Here's how the part is built. I have some questions about the finished solid (model axes, mm). A direction names the side the tool comes from. Give positions to 0.01 mm unless a question says otherwise; leave off trailing zeros. Write each loop counter-clockwise with the first axis right and the second up, starting at its lowest first coordinate (ties: lowest second). Pieces come first, ordered by that corner, then holes. Notation, with made-up numbers: (70.25, -38.5) - (86.25, -38.5) arc R27 ccw to (86.25, -2.5) - close; hole circle Ø1 at (89, 81). An arc over 180 degrees is marked (long way). Use one line per item in the form item = value. Start each with the question number.
Solid Edge part; units mm, degrees
sketch "Sketch1" plane through (0, 0, 0) normal (0, -1, 0) x (1, 0, 0)
  line L0 (0, 50) -> (4, 50)
  arc A0 (4, 50) -> (28, 78) centre (31.9985, 50.287) cw
  line L1 (28, 50) -> (28, 78)
  line L2 (28, 35) -> (28, 50)
  line L3 (152, 35) -> (28, 35)
  line L4 (152, 51) -> (152, 35)
  line L5 (180, 51) -> (152, 51)
  line L6 (180, 0) -> (180, 51)
  line L7 (0, 0) -> (180, 0)
  line L8 (0, 0) -> (0, 50)
extrude "Protrusion1" add sketch "Sketch1" against normal blind 70
sketch "Sketch2" plane through (180, 35, 25.5) normal (1, 0, 0) x (0, 1, 0)
  circle A0 centre (0, 25.5) radius 16
extrude "ExtrudedProtrusion_2" add sketch "Sketch2" against normal blind 28
sketch "Sketch3" plane through (180, 35, 33.5) normal (1, 0, 0) x (0, 1, 0)
  circle A0 centre (0, 17.5) radius 8
extrude "ExtrudedCutout_1" cut sketch "Sketch3" against normal blind 28 and the other way blind 1
sketch "Sketch4" plane through (180, 35, 33.5) normal (1, 0, 0) x (0, 1, 0)
  line L0 (16, -33.5) -> (16, -14.5)
  line L1 (16, -14.5) -> (8, -14.5)
  line L2 (8, -14.5) -> (8, 7.5)
  line L3 (8, 7.5) -> (-8, 7.5)
  line L4 (-8, 7.5) -> (-8, -14.5)
  line L5 (-8, -14.5) -> (-16, -14.5)
  line L6 (-16, -14.5) -> (-16, -33.5)
  line L7 (-16, -33.5) -> (16, -33.5)
extrude "ExtrudedCutout_2" cut sketch "Sketch4" against normal blind 180 and the other way blind 1
1. Please list where these lines run through material, in increasing order: line 1 (Z direction, x = 169, y = 35); line 2 (X direction, y = 63, z = 42); line 3 (X direction, y = 25, z = 51).
2. We'd pull the mould along X, two halves only. Please class faces 6 (the face through (91, 56, 35)), 7 (the face through (91, 13, 35)), 8 (the face through (166, 9, 51)), 9 (the face through (10.92, 34.51, 68.72)): pulls with the +X half, pulls with the -X half, needs draft (parallel to the pull), parting line crosses it, or undercut.
3. I want a section at B-B, the plane z = 27. List the corners of the cut face in (x, y) for me, then the cut area to 3 significant figures.
4. I want a section at C-C, the plane y = 35. List the corners of the cut face in (x, z) for me, then the cut area to 3 significant figures.
5. I want a section at D-D, the plane z = 39. List the corners of the cut face in (x, y) for me.
6. For faces 1 (the face through (91, 70, 21)), 2 (the face through (180, 26.7, 33)), 3 (the face through (166, 60, 51)), 4 (the face through (91, 23, 19)), 5 (the face through (166, 35, 67)), which set-ups out of +Z, -Z, +X, -X, +Y, -Y let a thin tool reach every point of the face, with its end or its side?
7. For P1, Ø3, axis at x = 1, y = 38.5, coming from the +Z side; P2, Ø8, axis at x = 10.5, y = 34, coming from the -Z side; P3, Ø21.5, axis at x = 86.5, y = 54, coming from the +Z side, each with a flat end and sliding along its axis, tell me the tip position at first contact or that it passes through.
8. I want a section at A-A, the plane x = 163.5. List the corners of the cut face in (y, z) for me.
Result sheet:
q1.line_1 = 41 to 43, 59 to 67
q1.line_2 = 0 to 28, 152 to 180
q1.line_3 = 4.01 to 28, 152 to 180
q2.face_6 = undercut
q2.face_7 = undercut
q2.face_8 = needs draft
q2.face_9 = pulls with the -X half
q3.outline = (0, 0) - (180, 0) - (180, 27) - (0, 27) - close; (0, 43) - (180, 43) - (180, 70) - (0, 70) - close
q3.area = 9,720 mm2
q4.outline = (0, 41) - (28, 41) - (28, 50) - (28, 78) arc R28 ccw to (4, 50) - (0, 50) - close; (152, 41) - (180, 41) - (180, 43) - (152, 43) - close; (152, 59) - (180, 59) - (180, 67) - (152, 67) - close
q4.area = 1,040 mm2
q5.outline = (0, 0) - (28, 0) - (28, 27) - (0, 27) - close; (0, 43) - (28, 43) - (28, 70) - (0, 70) - close; (152, 0) - (180, 0) - (180, 27) - (152, 27) - close; (152, 43) - (180, 43) - (180, 70) - (152, 70) - close
q6.face_1 = +Z, -Z, +X, -X, +Y
q6.face_2 = +Z, -Z, +X, +Y, -Y
q6.face_3 = +Z, +X, +Y
q6.face_4 = -Z, +X, -X
q6.face_5 = +Z, +X
q7.P1 = 50
q7.P2 = 41
q7.P3 = 35
q8.outline = (0, 0) - (19, 0) - (19, 19) - (27, 19) - (27, 41) - (43, 41) - (43, 19) - (51, 19) - (51, 0) - (70, 0) - (70, 51) - (51, 51) arc R16 ccw to (19, 51) - (0, 51) - close; hole circle Ø16 at (35, 51)
